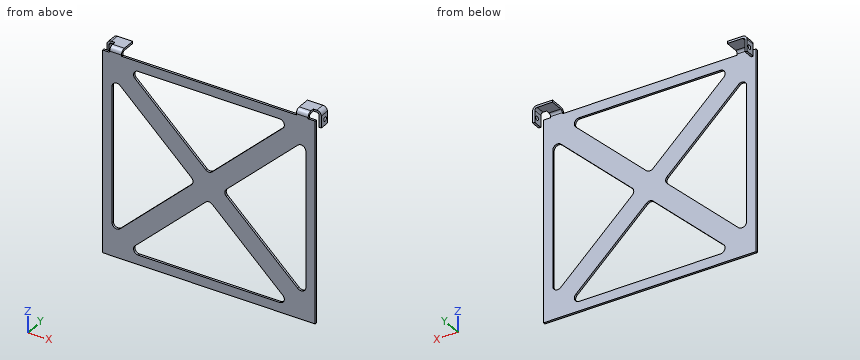
```python
from build123d import *

# Parameters (mm, degrees)
BOSS_EXTRUDE1_DEPTH                 = 1.5
SKETCH3_W                           = 5
SKETCH3_H                           = 1.5
BOSS_EXTRUDE2_DEPTH                 = 6.5
BOSS_EXTRUDE3_DEPTH                 = 6
BOSS_EXTRUDE3_DEPTH_BACK            = 1.5
SKETCH4_W                           = 1.5
SKETCH4_H                           = 4
BOSS_EXTRUDE3_2_DEPTH               = 6
BOSS_EXTRUDE3_2_DEPTH_BACK          = 1.5
SKETCH5_W                           = 2.5
SKETCH5_H                           = 1.5
BOSS_EXTRUDE4_DEPTH                 = 4
CONVERT_SOLID2_DEPTH                = 0.6
CONVERT_SOLID2_START                = 0.6
CONVERT_SOLID2_2_DEPTH              = 7.4
CONVERT_SOLID2_3_OUTLINE_W          = 5
CONVERT_SOLID2_3_OUTLINE_H          = 0.9
CONVERT_SOLID2_3_DEPTH              = 0.15504
CONVERT_SOLID2_START_2              = 4
CONVERT_SOLID2_4_DEPTH              = 4
CONVERT_SOLID2_START_3              = -42
CONVERT_SOLID2_5_DEPTH              = 84
CONVERT_SOLID2_6_DEPTH              = 5
CONVERT_SOLID2_START_4              = 37
CONVERT_SOLID2_7_DEPTH              = 5
F_0_CLEARANCE_HOLE1_D               = 1.778
F_0_CLEARANCE_HOLE1_DEPTH           = 3.175
F_0_CLEARANCE_HOLE1_TIP             = 0.53416509
F_0_CLEARANCE_HOLE1_ON_FACE_2_D     = 1.778
F_0_CLEARANCE_HOLE1_ON_FACE_2_DEPTH = 3.175
F_0_CLEARANCE_HOLE1_ON_FACE_2_TIP   = 0.53416509
CUT_EXTRUDE1_DEPTH                  = 65.182707952


with BuildPart() as part:
    # Sketch1 → Boss-Extrude1 (new body)
    with BuildSketch(Plane(origin=(0, 0, 0), x_dir=(1, 0, 0), z_dir=(0, 1, 0))):
        Polygon((-42, -45.5), (-42, -42.5), (-45, -42.5), (-45, 42.5), (45, 42.5), (45, -42.5), (42, -42.5), (42, -45.5), (37, -45.5), (37, -42.5), (-37, -42.5), (-37, -45.5), align=None)
    extrude(amount=BOSS_EXTRUDE1_DEPTH)

    # Sketch3 → Boss-Extrude2 (add)
    with BuildSketch(Plane(origin=(0, 1.5, 0), x_dir=(1, 0, 0), z_dir=(0, 1, 0))):
        with Locations((-39.5, -44.75)):
            Rectangle(SKETCH3_W, SKETCH3_H)
        with Locations((39.5, -44.75)):
            Rectangle(SKETCH3_W, SKETCH3_H)
    extrude(amount=BOSS_EXTRUDE2_DEPTH)



with BuildPart() as body_2:
    # Sketch4 → Boss-Extrude3 (new, two sides: drawn at the far end of the back side and taken through both)
    with BuildSketch(Plane(origin=(0, 0, 44), x_dir=(-1, 0, 0), z_dir=(0, 0, -1)).offset(-BOSS_EXTRUDE3_DEPTH_BACK)):
        with Locations((45.25, 6)):
            Rectangle(SKETCH4_W, SKETCH4_H)
    extrude(amount=BOSS_EXTRUDE3_DEPTH + BOSS_EXTRUDE3_DEPTH_BACK)


with BuildPart() as body_3:
    # Sketch4 → Boss-Extrude3 2 (new, two sides: drawn at the far end of the back side and taken through both)
    with BuildSketch(Plane(origin=(0, 0, 44), x_dir=(-1, 0, 0), z_dir=(0, 0, -1)).offset(-BOSS_EXTRUDE3_2_DEPTH_BACK)):
        with Locations((-45.25, 6)):
            Rectangle(SKETCH4_W, SKETCH4_H)
    extrude(amount=BOSS_EXTRUDE3_2_DEPTH + BOSS_EXTRUDE3_2_DEPTH_BACK)


with BuildPart() as part_1:
    add(part.part)

    add(body_2.part)  # Boss-Extrude4 merges body 2

    add(body_3.part)  # Boss-Extrude4 merges body 3
    # Sketch5 → Boss-Extrude4 (add)
    with BuildSketch(Plane(origin=(0, 8, 0), x_dir=(1, 0, 0), z_dir=(0, 1, 0))):
        with Locations((-43.25, -44.75)):
            Rectangle(SKETCH5_W, SKETCH5_H)
        with Locations((43.25, -44.75)):
            Rectangle(SKETCH5_W, SKETCH5_H)
    extrude(amount=-BOSS_EXTRUDE4_DEPTH)

    # Convert-Solid2: read off the stored shape, not the designer's step
    # Convert-Solid2 outline → Convert-Solid2 (cut)
    with BuildSketch(Plane(origin=(0, 0, 0), x_dir=(1, 0, 0), z_dir=(0, 1, 0))):
        Polygon((37, -45.5), (42, -45.5), (42, -42.5), (45, -42.5), (45, 42.5), (-45, 42.5), (-45, -42.5), (-42, -42.5), (-42, -45.5), (-37, -45.5), (-37, -42.5), (37, -42.5), align=None)
    extrude(amount=CONVERT_SOLID2_DEPTH, mode=Mode.SUBTRACT)

    # Convert-Solid2 2 outline → Convert-Solid2 2 (cut)
    with BuildSketch(Plane(origin=(0, 0, 0), x_dir=(1, 0, 0), z_dir=(0, 1, 0)).offset(CONVERT_SOLID2_START)):
        with BuildLine():
            Line((37, -45.5), (46, -45.5))
            Line((46, -45.5), (46, -38))
            Line((46, -38), (45.4, -38))
            Line((45.4, -38), (45.4, -43))
            ThreePointArc((45.4, -43), (44.843502884, -44.343502884), (43.5, -44.9))
            Line((43.5, -44.9), (37, -44.9))
            Line((37, -44.9), (37, -45.5))
        make_face()
        with BuildLine():
            Line((-37, -45.5), (-37, -44.9))
            Line((-37, -44.9), (-43.5, -44.9))
            ThreePointArc((-43.5, -44.9), (-44.843502884, -44.343502884), (-45.4, -43))
            Line((-45.4, -43), (-45.4, -38))
            Line((-45.4, -38), (-46, -38))
            Line((-46, -38), (-46, -45.5))
            Line((-46, -45.5), (-37, -45.5))
        make_face()
    extrude(amount=CONVERT_SOLID2_2_DEPTH, mode=Mode.SUBTRACT)

    # Convert-Solid2 3 outline → Convert-Solid2 3 (cut)
    with BuildSketch(Plane(origin=(0, 0, 0), x_dir=(1, 0, 0), z_dir=(0, 1, 0)).offset(CONVERT_SOLID2_START)):
        with Locations((39.5, -44.45)):
            Rectangle(CONVERT_SOLID2_3_OUTLINE_W, CONVERT_SOLID2_3_OUTLINE_H)
        with Locations((-39.5, -44.45)):
            Rectangle(CONVERT_SOLID2_3_OUTLINE_W, CONVERT_SOLID2_3_OUTLINE_H)
    extrude(amount=CONVERT_SOLID2_3_DEPTH, mode=Mode.SUBTRACT)

    # Convert-Solid2 4 outline → Convert-Solid2 4 (add)
    with BuildSketch(Plane(origin=(0, 0, 0), x_dir=(1, 0, 0), z_dir=(0, 1, 0)).offset(CONVERT_SOLID2_START_2)):
        with BuildLine():
            ThreePointArc((44.5, -43), (44.207106781, -43.707106781), (43.5, -44))
            Line((43.5, -44), (44.5, -44))
            Line((44.5, -44), (44.5, -43))
        make_face()
        with BuildLine():
            Line((-44.5, -44), (-43.5, -44))
            ThreePointArc((-43.5, -44), (-44.207106781, -43.707106781), (-44.5, -43))
            Line((-44.5, -43), (-44.5, -44))
        make_face()
    extrude(amount=CONVERT_SOLID2_4_DEPTH)

    # Convert-Solid2 5 outline → Convert-Solid2 5 (cut)
    with BuildSketch(Plane.YZ.offset(CONVERT_SOLID2_START_3)):
        with BuildLine():
            ThreePointArc((0.6, 43), (1.156497116, 44.343502884), (2.5, 44.9))
            Line((2.5, 44.9), (0.75504, 44.9))
            Line((0.75504, 44.9), (0.75504, 44))
            Line((0.75504, 44), (0.6, 44))
            Line((0.6, 44), (0.6, 43))
        make_face()
    extrude(amount=CONVERT_SOLID2_5_DEPTH, mode=Mode.SUBTRACT)

    # Convert-Solid2 6 outline → Convert-Solid2 6 (add)
    with BuildSketch(Plane.YZ.offset(CONVERT_SOLID2_START_3)):
        with BuildLine():
            ThreePointArc((1.5, 43), (1.792893219, 43.707106781), (2.5, 44))
            Line((2.5, 44), (1.5, 44))
            Line((1.5, 44), (1.5, 43))
        make_face()
    extrude(amount=CONVERT_SOLID2_6_DEPTH)

    # Convert-Solid2 7 outline → Convert-Solid2 7 (add)
    with BuildSketch(Plane.YZ.offset(CONVERT_SOLID2_START_4)):
        with BuildLine():
            ThreePointArc((1.5, 43), (1.792893219, 43.707106781), (2.5, 44))
            Line((2.5, 44), (1.5, 44))
            Line((1.5, 44), (1.5, 43))
        make_face()
    extrude(amount=CONVERT_SOLID2_7_DEPTH)

    # #0 Clearance Hole1
    with Locations(Plane(origin=(-44.5, 6.5, 40.5), x_dir=(0, 0, 1), z_dir=(1, 0, 0))):
        with Locations((0, 0)):
            Hole(F_0_CLEARANCE_HOLE1_D / 2, depth=F_0_CLEARANCE_HOLE1_DEPTH)
            with Locations((0, 0, -(F_0_CLEARANCE_HOLE1_DEPTH + F_0_CLEARANCE_HOLE1_TIP / 2))):  # 118° drill point
                Cone(0, F_0_CLEARANCE_HOLE1_D / 2, F_0_CLEARANCE_HOLE1_TIP, mode=Mode.SUBTRACT)

    # #0 Clearance Hole1 on face 2
    with Locations(Plane(origin=(44.5, 6.5, 40.5), x_dir=(0, 0, -1), z_dir=(-1, 0, 0))):
        with Locations((0, 0)):
            Hole(F_0_CLEARANCE_HOLE1_ON_FACE_2_D / 2, depth=F_0_CLEARANCE_HOLE1_ON_FACE_2_DEPTH)
            with Locations((0, 0, -(F_0_CLEARANCE_HOLE1_ON_FACE_2_DEPTH + F_0_CLEARANCE_HOLE1_ON_FACE_2_TIP / 2))):  # 118° drill point
                Cone(0, F_0_CLEARANCE_HOLE1_ON_FACE_2_D / 2, F_0_CLEARANCE_HOLE1_ON_FACE_2_TIP, mode=Mode.SUBTRACT)

    # Sketch18 → Cut-Extrude1 (cut, through all)
    with BuildSketch(Plane(origin=(0, 1.5, 0), x_dir=(1, 0, 0), z_dir=(0, 1, 0))):
        with BuildLine():
            Line((-1.373247066, -6.798919297), (-31.281892899, -35.045973695))
            ThreePointArc((-31.281892899, -35.045973695), (-31.767146924, -37.238900328), (-29.908645833, -38.5))
            Line((-29.908645833, -38.5), (29.908645833, -38.5))
            ThreePointArc((29.908645833, -38.5), (31.767146924, -37.238900328), (31.281892899, -35.045973695))
            Line((31.281892899, -35.045973695), (1.373247066, -6.798919297))
            ThreePointArc((1.373247066, -6.798919297), (0, -6.252945602), (-1.373247066, -6.798919297))
        make_face()
        with BuildLine():
            Line((-7.365165925, 1.454026305), (-37.626752934, 30.034414036))
            ThreePointArc((-37.626752934, 30.034414036), (-39.791677292, 30.417027888), (-41, 28.580387731))
            Line((-41, 28.580387731), (-41, -28.580387731))
            ThreePointArc((-41, -28.580387731), (-39.791677292, -30.417027888), (-37.626752934, -30.034414036))
            Line((-37.626752934, -30.034414036), (-7.365165925, -1.454026305))
            ThreePointArc((-7.365165925, -1.454026305), (-6.73841299, 0), (-7.365165925, 1.454026305))
        make_face()
        with BuildLine():
            Line((7.365165925, 1.454026305), (37.626752934, 30.034414036))
            ThreePointArc((37.626752934, 30.034414036), (39.791677292, 30.417027888), (41, 28.580387731))
            Line((41, 28.580387731), (41, -28.580387731))
            ThreePointArc((41, -28.580387731), (39.791677292, -30.417027888), (37.626752934, -30.034414036))
            Line((37.626752934, -30.034414036), (7.365165925, -1.454026305))
            ThreePointArc((7.365165925, -1.454026305), (6.73841299, 0), (7.365165925, 1.454026305))
        make_face()
        with BuildLine():
            Line((-31.281892899, 35.045973695), (-1.373247066, 6.798919297))
            ThreePointArc((-1.373247066, 6.798919297), (0, 6.252945602), (1.373247066, 6.798919297))
            Line((1.373247066, 6.798919297), (31.281892899, 35.045973695))
            ThreePointArc((31.281892899, 35.045973695), (31.767146924, 37.238900328), (29.908645833, 38.5))
            Line((29.908645833, 38.5), (-29.908645833, 38.5))
            ThreePointArc((-29.908645833, 38.5), (-31.767146924, 37.238900328), (-31.281892899, 35.045973695))
        make_face()
    extrude(amount=-CUT_EXTRUDE1_DEPTH, mode=Mode.SUBTRACT)


solid = part_1.part
```
Check sheet for the modelled part. Datum: model origin and axes. Units: mm. Give positions to 0.01 mm unless a question says otherwise; leave off trailing zeros. Write each loop counter-clockwise with the first axis right and the second up, starting at its lowest first coordinate (ties: lowest second). Pieces come first, ordered by that corner, then holes. Notation, with made-up numbers: (79.25, 18.25) - (85.25, 18.25) arc R16 cw to (85.25, 38.25) - close; hole circle Ø6 at (63, -7.5). An arc over 180 degrees is marked (long way). Answer as a JSON object with one key per item and string values. Group by question number.
1) Depth check by flat-ended pin: P1, Ø0.7, axis at y = 2, z = 43.5, coming from the -X side; P2, Ø1, axis at y = 1, z = -8.5, coming from the -X side; P3, Ø0.7, axis at x = -2.5, y = 1, coming from the +Z side. Enter the tip coordinate at first touch or a pass-through.
2) Sectioned sample at A-A (x = 25.5). Record the cut outline in (y, z).
3) Sectioned sample at B-B (z = 10). Record the cut outline in (x, y), then the cut area to 3 significant figures.
4) Thickness scan on probe 1 along Y at (x, z) = (-44.9, 40.5); probe 2 along Y at (x, z) = (-45.05, 40.5); probe 3 along Y at (x, z) = (5, 9). Record the ranges inside material, lowest first. Write a range as from..to.
5) Sectioned sample at C-C (x = -34). Record the cut outline in (y, z), then the cut area to 3 significant figures.
Geometry results:
{
 "1": {"P1": "stops at x = -42", "P2": "stops at x = -45", "P3": "stops at z = 42.5"},
 "2": {"outline": "(0.6, -42.5) - (1.5, -42.5) - (1.5, -38.5) - (0.6, -38.5) - close; (0.6, -29.59) - (1.5, -29.59) - (1.5, -18.58) - (0.6, -18.58) - close; (0.6, 18.58) - (1.5, 18.58) - (1.5, 29.59) - (0.6, 29.59) - close; (0.6, 38.5) - (1.5, 38.5) - (1.5, 42.5) - (0.6, 42.5) - close"},
 "3": {"outline": "(-45, 0.6) - (-41, 0.6) - (-41, 1.5) - (-45, 1.5) - close; (-16.41, 0.6) - (-4.76, 0.6) - (-4.76, 1.5) - (-16.41, 1.5) - close; (4.76, 0.6) - (16.41, 0.6) - (16.41, 1.5) - (4.76, 1.5) - close; (41, 0.6) - (45, 0.6) - (45, 1.5) - (41, 1.5) - close", "area": "28.2 mm^2"},
 "4": {"probe 1": "y = 0.6..1.5, 4..5.61, 7.39..8", "probe 2": "y = 4..5.61, 7.39..8", "probe 3": "y = 0.6..1.5"},
 "5": {"outline": "(0.6, -42.5) - (1.5, -42.5) - (1.5, -26.61) - (0.6, -26.61) - close; (0.6, 26.61) - (1.5, 26.61) - (1.5, 42.5) - (0.6, 42.5) - close", "area": "28.6 mm^2"}
}
